Can you work these out from the drawing? Everything is in mm from the part's minimum corner. A direction names the side the tool comes from. Round coordinates to 2 decimals unless told otherwise and drop trailing zeros. Loops run counter-clockwise (first coordinate to the right, second up) from the corner with the lowest first, then second, coordinate; pieces in that order, holes last. Notation, with made-up numbers: M 16.25,43 L 50.25,43 A7 ccw 50.25,55 Z; hole C 32.5,-32 d5. An arc over 180 degrees is marked long. Answer in a Markdown table with one row per item.
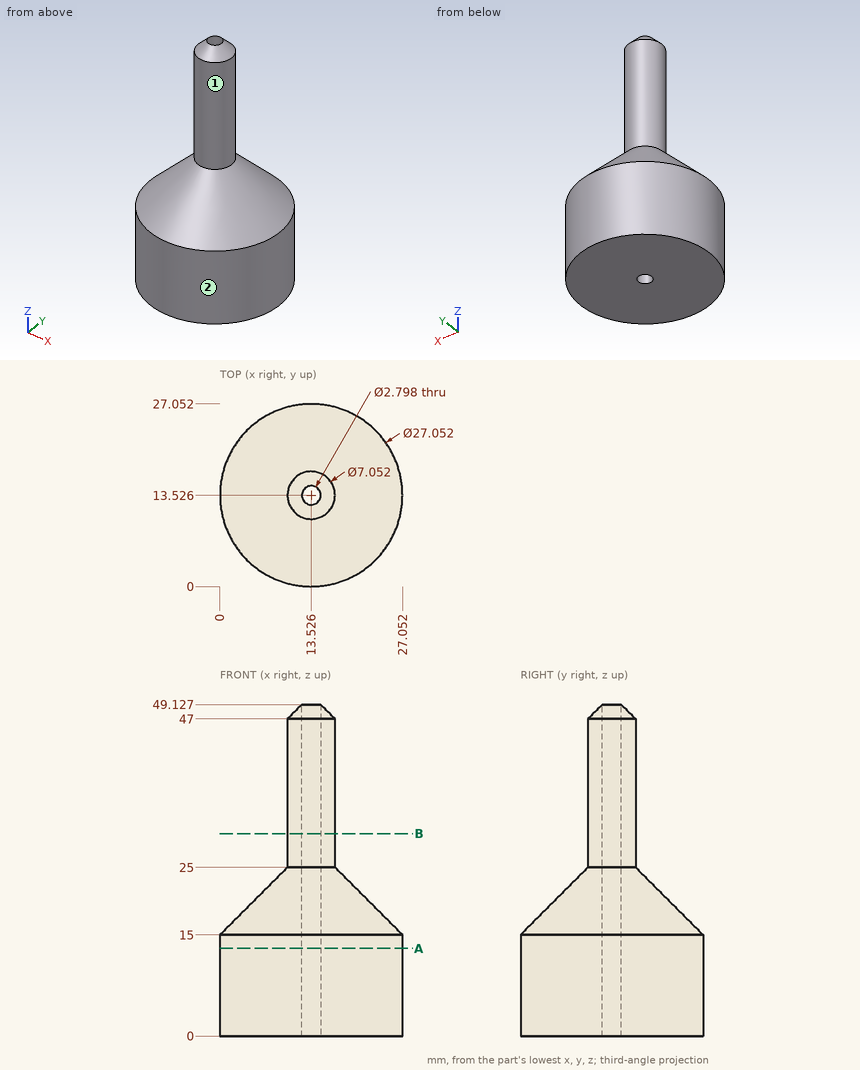
1) Which directions (+Z, -Z, +X, -X, +Y, -Y) give clear straight access to the entire face, cutting with the end or side of a thin tool? Please do the marked faces 1 and 2.
Computed:
| item | result |
|---|---|
| face 1 | +Z |
| face 2 | +Z, -Z |
2) I want a section at B-B, the plane z = 30. Please give me the cut outline in (x, y) (1 decimal).
Computed:
| item | result |
|---|---|
| outline | C 13.5,13.5 d7.1; hole C 13.5,13.5 d2.8 |
3) I want a section at A-A, the plane z = 13. Please give me the cut outline in (x, y) (1 decimal).
Computed:
| item | result |
|---|---|
| outline | C 13.5,13.5 d27.1; hole C 13.5,13.5 d2.8 |
4) I need wall thicknesses on line 1 (X direction, y = 12.75, z = 37) (1 decimal); line 2 (Y direction, x = 14.5, z = 42.5) (1 decimal). Which ranges of each line are inside material? Lowest first, please.
Computed:
| item | result |
|---|---|
| line 1 | x = 10.1 to 12.4, 14.7 to 17 |
| line 2 | y = 10.1 to 12.5, 14.5 to 16.9 |
5) Will these pins go through, and if not, where does the flat tip stop? P1, Ø10, axis at x = 10, z = 39, coming from the +Y side; P2, Ø10, axis at x = 4, y = 22.5, coming from the +Z side; P3, Ø2, axis at y = 11.5, z = 35.5, coming from the +X side.
Computed:
| item | result |
|---|---|
| P1 | stops at y = 17.05 |
| P2 | stops at z = 20.44 |
| P3 | stops at x = 16.9 |
